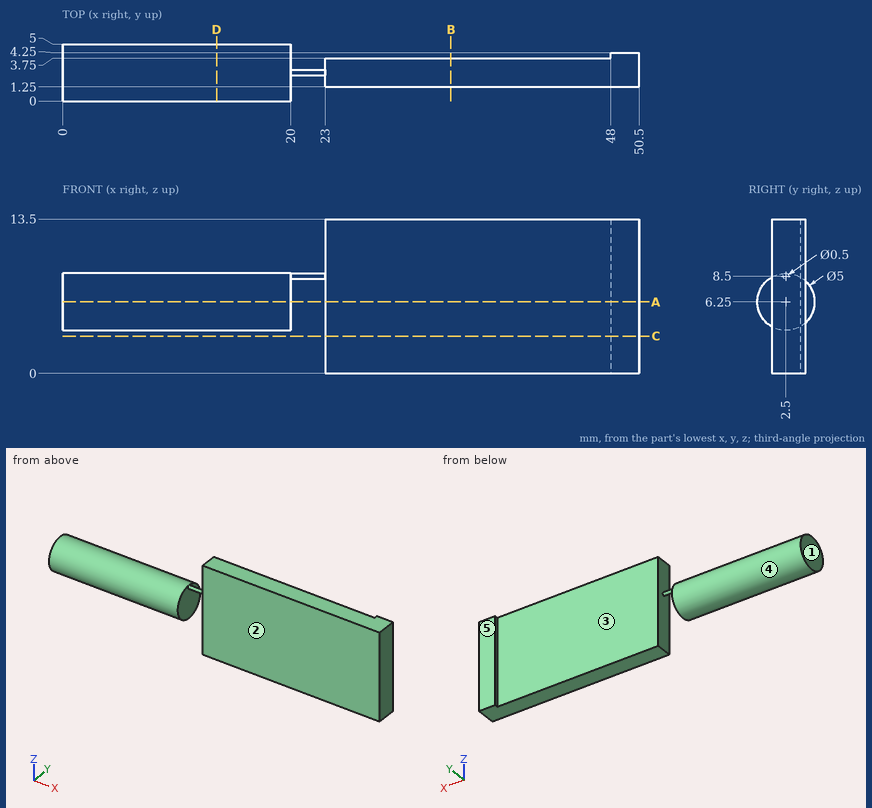
Geometry check sheet. Reference: drawing and pictorial views, mm from the part's lowest x, y, z. A direction names the side the tool comes from. Round coordinates to 2 decimals unless told otherwise and drop trailing zeros. Write each loop counter-clockwise with the first axis right and the second up, starting at its lowest first coordinate (ties: lowest second). Pieces come first, ordered by that corner, then holes.
Item 1: Mould release check, pull along X, two halves, no side actions. Record for the marked faces 1, 2 and 3: +X half, -X half, draft (parallel to the pull), parting line (faces both ways), or undercut.
Determined:
face 1: -X half
face 2: draft
face 3: undercut
Item 2: Section check C-C (z = 3.25). Record the boundary of the cut face in (x, y), plus the area to 3 significant figures.
Determined:
outline: (23, 1.25) - (50.5, 1.25) - (50.5, 4.25) - (48, 4.25) - (48, 3.75) - (23, 3.75) - close
area: 70.0 mm2
Item 3: Section check B-B (x = 34). Record the boundary of the cut face in (y, z), plus the area to 4 significant figures.
Determined:
outline: (1.25, 0) - (3.75, 0) - (3.75, 13.5) - (1.25, 13.5) - close
area: 33.75 mm2
Item 4: Material ranges on line 1 along X through (y, z) = (2.3, 7); line 2 along X through (y, z) = (1.3, 9); line 3 along X through (y, z) = (4.3, 6), recorded low to high.
Determined:
line 1: x = 0 to 20, 23 to 50.5
line 2: x = 23 to 50.5
line 3: x = 0 to 20
Item 5: Access from +Z, -Z, +X, -X, +Y, -Y to the whole of each face (thin tool, end or side, straight path). Record for the marked faces 4 and 5.
Determined:
face 4: -X
face 5: +Z, -Z, +X, +Y
Item 6: Section check A-A (z = 6.25). Record the boundary of the cut face in (x, y).
Determined:
outline: (0, 0) - (20, 0) - (20, 5) - (0, 5) - close; (23, 1.25) - (50.5, 1.25) - (50.5, 4.25) - (48, 4.25) - (48, 3.75) - (23, 3.75) - close
Item 7: Section check D-D (x = 13.5). Record the boundary of the cut face in (y, z), plus the area to 3 significant figures.
Determined:
outline: circle Ø5 at (2.5, 6.25)
area: 19.6 mm2
Item 8: Go/stop test with flat-tipped pins: pin 1 Ø2 at (x, z) = (50, 7) entering from +Y; pin 2 Ø7 at (x, z) = (32.5, 10) entering from +Y; pin 3 Ø1 at (y, z) = (0.5, 2.5) entering from +X; pin 4 Ø2 at (y, z) = (0.5, 5) entering from -X. Record where each tip stops, or that it passes through.
Determined:
pin 1: stops at y = 4.25
pin 2: stops at y = 3.75
pin 3: passes through
pin 4: stops at x = 0
